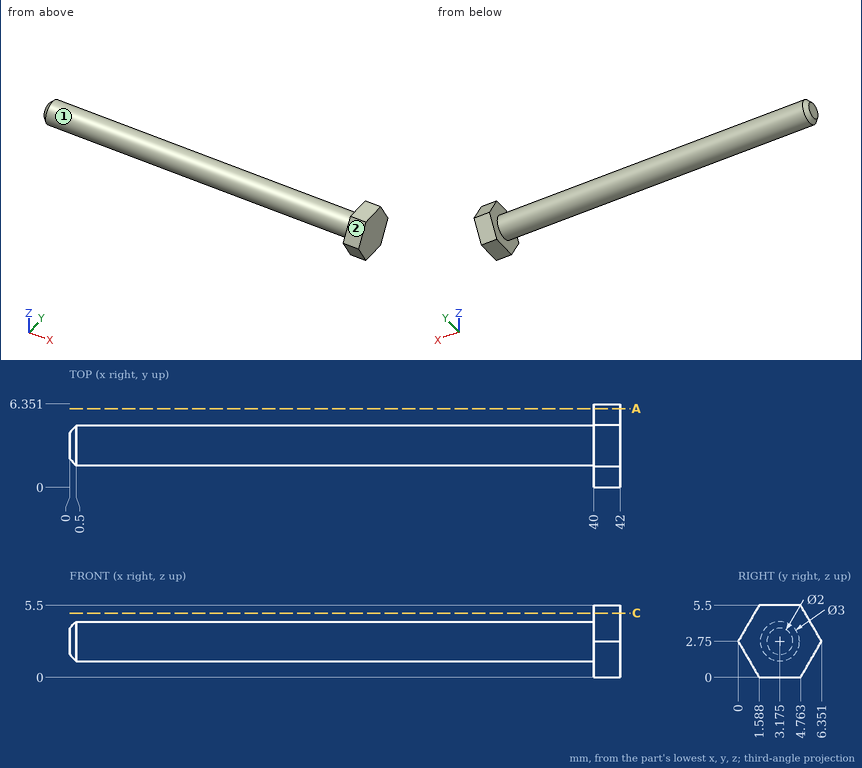
Geometry check sheet. Reference: drawing and pictorial views, mm from the part's lowest x, y, z. A direction names the side the tool comes from. Round coordinates to 2 decimals unless told otherwise and drop trailing zeros. Order: outer loops, then holes, each group sorted by start corner. A loop starts at its lowest first (then second) coordinate and runs counter-clockwise, first axis right, second up. Notation, with made-up numbers: (-18, 52.5) - (12, 52.5) arc R29 ccw to (12, 73.5) - close; hole circle Ø5 at (-28.75, -8). An arc over 180 degrees is marked (long way). One line per question, with ' | ' between items. Start each with the question number.
(1) Sectioned sample at C-C on z = 4.9. Record the cut outline in (x, y).
(2) Sectioned sample at A-A on y = 6. Record the cut outline in (x, z).
(3) Access from +Z, -Z, +X, -X, +Y, -Y to the whole of each face (thin tool, end or side, straight path). Record for the marked faces 1 and 2.
(4) Depth check by flat-ended pin: pin 1 Ø1 at (x, z) = (37, 3.5) entering from -Y; pin 2 Ø2 at (x, y) = (35, 2.5) entering from +Z; pin 3 Ø2 at (x, y) = (14.5, 5.5) entering from +Z (1 decimal); pin 4 Ø1.6 at (y, z) = (3, 2.5) entering from -X. Enter the tip coordinate at first touch or a pass-through.
(5) Thickness scan on L1, parallel to X at y = 1.25, z = 3.95; L2, parallel to Y at x = 12.5, z = 2.65; L3, parallel to Z at x = 27.5, y = 3.25. Record the ranges inside material, lowest first. Write a range as [from, to].
Conclusion:
1) outline: (40, 1.24) - (42, 1.24) - (42, 5.11) - (40, 5.11) - close
2) outline: (40, 2.14) - (42, 2.14) - (42, 3.36) - (40, 3.36) - close
3) face 1: -X | face 2: +Z, +X, -X, -Y
4) pin 1: stops at y = 1.7 | pin 2: stops at z = 4.25 | pin 3: stops at z = 3.5 | pin 4: stops at x = 0
5) L1: x = [40, 42] | L2: y = [1.68, 4.67] | L3: z = [1.25, 4.25]
